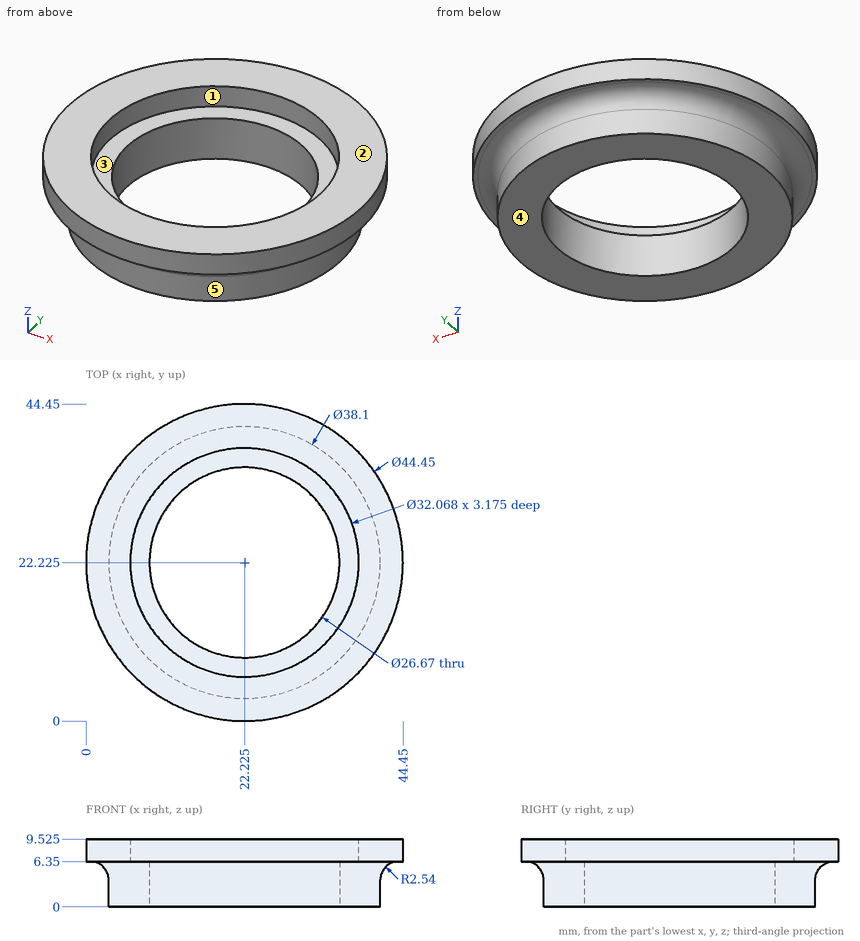
Could you check a few things on this drawing? It's one solid part, dimensions in mm from its lowest x, y, z. A direction names the side the tool comes from. Round coordinates to 2 decimals unless told otherwise and drop trailing zeros. Answer as CSV lines item,"result".
1. For pin 1 (12 mm diameter, centred on x = 30, y = 20, fed in from +Z); pin 2 (19 mm diameter, centred on x = 22.225, y = 22.225, fed in from +Z); pin 3 (4 mm diameter, centred on x = 13.5, z = 3.5, fed in from +Y) (1 decimal); pin 4 (1 mm diameter, centred on y = 32, z = 2.5, fed in from +X) (1 decimal), each with a flat end and sliding along its axis, tell me the tip position at first contact or that it passes through.
Final values:
pin 1,"stops at z = 6.35"
pin 2,"passes through"
pin 3,"stops at y = 40.1"
pin 4,"stops at x = 38.9"
2. Thinking about a two-plate mould opening in X: for the marked faces 3, 4 and 5, which applies, released by +X, released by -X, zero draft, split by the parting line, or undercut?
Final values:
face 3,"undercut"
face 4,"zero draft"
face 5,"split by the parting line"
3. Which directions (+Z, -Z, +X, -X, +Y, -Y) give clear straight access to the entire face, cutting with the end or side of a thin tool? Please do the marked faces 1 and 2.
Final values:
face 1,"+Z"
face 2,"+Z, +X, -X, +Y, -Y"
4. If I drill on L1, parallel to Y at x = 22.5, z = 7.75; L2, parallel to X at y = 11, z = 5.75 (1 decimal); L3, parallel to Y at x = 12, z = 8.75 (1 decimal), over which ranges is the centre line in solid material (lowest first)?
Final values:
L1,"y = 0 to 6.19, 38.26 to 44.45"
L2,"x = 5.7 to 15, 29.4 to 38.7"
L3,"y = 2.5 to 9.9, 34.6 to 42"
